```python
from build123d import *

# Parameters (mm, degrees)
F3_DEPTH = 10


with BuildPart() as f1:
    # F0 (on Right) → F1 (revolve)
    with BuildSketch(Plane.YZ):
        Polygon((-14, 3.431979), (0, 3.431979), (0, 25.684212), (-6, 25.684212), (-6, 19.684212), (-14, 19.684212), align=None)
    revolve(axis=Axis((0, -7, 0), (0, 1, 0)))

    # F2 (on face) → F3 (join)
    with BuildSketch(Plane.XZ.offset(14)):
        Polygon((-10.437276, -19.684212), (0, -19.684212), (11.577706, -19.684212), (11.577706, -19.137302), (-10.437276, -19.137302), align=None)
    extrude(amount=-F3_DEPTH)


solid = f1.part
```
Check sheet for the modelled part. Datum: model origin and axes. Units: mm. Round coordinates to 2 decimals unless told otherwise and drop trailing zeros. Loops run counter-clockwise (first coordinate to the right, second up) from the corner with the lowest first, then second, coordinate; pieces in that order, holes last. Notation, with made-up numbers: M -13.5,-30 L 34.5,-30 A12 cw 34.5,-20 Z; hole C -18.5,54.5 d11. An arc over 180 degrees is marked long. Answer as a JSON object with one key per item and string values.
1. Section check D-D (z = 12.5). Record the boundary of the cut face in (x, y), plus the area to 3 significant figures.
Reply:
{"outline": "M -22.44,-6 L -15.21,-6 L -15.21,-14 L 15.21,-14 L 15.21,-6 L 22.44,-6 L 22.44,0 L -22.44,0 Z", "area": "513 mm²"}
2. Section check A-A (z = 0). Record the boundary of the cut face in (x, y).
Reply:
{"outline": "M -25.68,-6 L -19.68,-6 L -19.68,-14 L -3.43,-14 L -3.43,0 L -25.68,0 Z; M 3.43,-14 L 19.68,-14 L 19.68,-6 L 25.68,-6 L 25.68,0 L 3.43,0 Z"}
3. Scan lines: line 1 (X direction, y = -2.75, z = 0); line 2 (X direction, y = -6.25, z = 0); line 3 (Y direction, x = -10, z = 20.5). Record each from-to range of solid material in increasing order.
Reply:
{"line 1": "x = -25.68 to -3.43, 3.43 to 25.68", "line 2": "x = -19.68 to -3.43, 3.43 to 19.68", "line 3": "y = -6 to 0"}
4. Section check B-B (x = 0). Record the boundary of the cut face in (y, z).
Reply:
{"outline": "M -14,-19.68 L -6,-19.68 L -6,-25.68 L 0,-25.68 L 0,-3.43 L -14,-3.43 Z; M -14,3.43 L 0,3.43 L 0,25.68 L -6,25.68 L -6,19.68 L -14,19.68 Z"}
5. Section check C-C (y = -8.5). Record the boundary of the cut face in (x, z).
Reply:
{"outline": "M -10.44,-19.68 L 11.58,-19.68 L 11.58,-19.14 L 4.61,-19.14 A19.68 ccw long -4.61,-19.14 L -10.44,-19.14 Z; hole C 0,0 d6.86"}
6. Gauge pin test, flat ends, axial feed: P1, Ø4, axis at y = -10.5, z = -13, coming from the -X side; P2, Ø2, axis at x = 8.5, y = -10.5, coming from the +Z side; P3, Ø6.5, axis at x = -7, y = -11, coming from the +Z side. Record the tip position at first contact, or that the pin passes through.
Reply:
{"P1": "stops at x = -16.32", "P2": "stops at z = 18.2", "P3": "stops at z = 19.32"}
7. Mould release check, pull along Z, two halves, no side actions. Record for faces 1 (the flat face through (-5, 0, 0)), 2 (the flat face through (0, -10, -19.684)), 3 (the flat face through (8, -10, -19.137)): pulls with the +Z half, pulls with the -Z half, needs draft (parallel to the pull), parting line crosses it, or undercut.
Reply:
{"face 1": "needs draft", "face 2": "pulls with the -Z half", "face 3": "undercut"}
